```python
from build123d import *

# Parameters (mm, degrees)
F0_W     = 1016
F0_H     = 611.1875
F0_W_2   = 5.08
F0_H_2   = 5.08
F0_W_3   = 990.6
F0_H_3   = 585.7875
F0_R     = 5.969
F0_W_4   = 951.992
F0_H_4   = 552.45
F0_W_5   = 923.392
F0_H_5   = 523.85
F1_DEPTH = 1.5875


# Not quite as in the source:
# - a feature names something its author has since deleted; it is built from what else it names


with BuildPart() as f1:
    # F0 (on Front) → F1 (new body, symmetric)
    with BuildSketch(Plane.XZ):
        Rectangle(F0_W, F0_H)
        with Locations((-488.95, -299.24375)):
            Rectangle(F0_W_2, F0_H_2, mode=Mode.SUBTRACT)
        Polygon((-504.19, -284.00375), (-501.65, -284.00375), (-499.11, -284.00375), (-499.11, -289.08375), (-504.19, -289.08375), align=None, mode=Mode.SUBTRACT)
        with Locations((-357.84, -299.24375)):
            Rectangle(F0_W_2, F0_H_2, mode=Mode.SUBTRACT)
        Polygon((-504.19, -92.9745833333), (-501.65, -92.9745833333), (-499.11, -92.9745833333), (-499.11, -98.0545833333), (-501.65, -98.0545833333), (-504.19, -98.0545833333), align=None, mode=Mode.SUBTRACT)
        with Locations((357.84, -299.24375)):
            Rectangle(F0_W_2, F0_H_2, mode=Mode.SUBTRACT)
        with Locations((488.95, -299.24375)):
            Rectangle(F0_W_2, F0_H_2, mode=Mode.SUBTRACT)
        with Locations((501.65, -286.54375)):
            Rectangle(F0_W_2, F0_H_2, mode=Mode.SUBTRACT)
        Rectangle(F0_W_3, F0_H_3, mode=Mode.SUBTRACT)
        with Locations((501.65, -95.5145833333)):
            Rectangle(F0_W_2, F0_H_2, mode=Mode.SUBTRACT)
        Polygon((-504.19, 98.0545833333), (-501.65, 98.0545833333), (-499.11, 98.0545833333), (-499.11, 92.9745833333), (-501.65, 92.9745833333), (-504.19, 92.9745833333), align=None, mode=Mode.SUBTRACT)
        Polygon((-501.65, 284.00375), (-504.19, 284.00375), (-504.19, 289.08375), (-499.11, 289.08375), (-499.11, 284.00375), align=None, mode=Mode.SUBTRACT)
        with Locations((-488.95, 299.24375)):
            Circle(F0_R, mode=Mode.SUBTRACT)
        with Locations((-244.475, 299.24375)):
            Rectangle(F0_W_2, F0_H_2, mode=Mode.SUBTRACT)
        with Locations((501.65, 95.5145833333)):
            Rectangle(F0_W_2, F0_H_2, mode=Mode.SUBTRACT)
        with Locations((0, 299.24375)):
            Rectangle(F0_W_2, F0_H_2, mode=Mode.SUBTRACT)
        with Locations((244.475, 299.24375)):
            Rectangle(F0_W_2, F0_H_2, mode=Mode.SUBTRACT)
        with Locations((501.65, 286.54375)):
            Rectangle(F0_W_2, F0_H_2, mode=Mode.SUBTRACT)
        with Locations((488.95, 299.24375)):
            Rectangle(F0_W_2, F0_H_2, mode=Mode.SUBTRACT)
        Rectangle(F0_W_3, F0_H_3)
        Rectangle(F0_W_4, F0_H_4, mode=Mode.SUBTRACT)
        Rectangle(F0_W_4, F0_H_4)
        Rectangle(F0_W_5, F0_H_5, mode=Mode.SUBTRACT)
        with Locations((-488.95, 299.24375)):
            Circle(F0_R)
        with Locations((-488.95, 299.24375)):
            Rectangle(F0_W_2, F0_H_2, mode=Mode.SUBTRACT)
    extrude(amount=F1_DEPTH, both=True)


solid = f1.part
```
The model under review builds one solid part; all positions refer to its coordinate system, in mm. Round coordinates to 2 decimals unless told otherwise and drop trailing zeros. Loops run counter-clockwise (first coordinate to the right, second up) from the corner with the lowest first, then second, coordinate; pieces in that order, holes last.
Item 1: For line 1 (X direction, y = 1.45, z = -96); line 2 (Z direction, x = -452, y = -0.6) (3 decimals); line 3 (X direction, y = 1.5, z = -236.5), list the stretches that pass through material, from the lowest coordinate up.
Determined:
line 1: x = -508 to -504.19, -499.11 to -461.7, 461.7 to 499.11, 504.19 to 508
line 2: z = -305.594 to -261.925, 261.925 to 305.594
line 3: x = -508 to -461.7, 461.7 to 508
Item 2: Take a section at C-C (y = -0.3). Give the number of separate pieces and of enclosed holes in the cut face, then the cut area to 3 significant figures.
Determined:
separate pieces: 1
enclosed holes: 18
area: 137,000 mm2
Item 3: Take a section at B-B (x = -170). Write out the cut boundary in (y, z) (1 decimal), then the cut area to 3 significant figures.
Determined:
outline: (-1.6, -305.6) - (1.6, -305.6) - (1.6, -261.9) - (-1.6, -261.9) - close; (-1.6, 261.9) - (1.6, 261.9) - (1.6, 305.6) - (-1.6, 305.6) - close
area: 277 mm2
Item 4: Take a section at A-A (z = 12). Write out the cut boundary in (x, y), then the cut area to 3 significant figures.
Determined:
outline: (-508, -1.59) - (-461.7, -1.59) - (-461.7, 1.59) - (-508, 1.59) - close; (461.7, -1.59) - (508, -1.59) - (508, 1.59) - (461.7, 1.59) - close
area: 294 mm2
